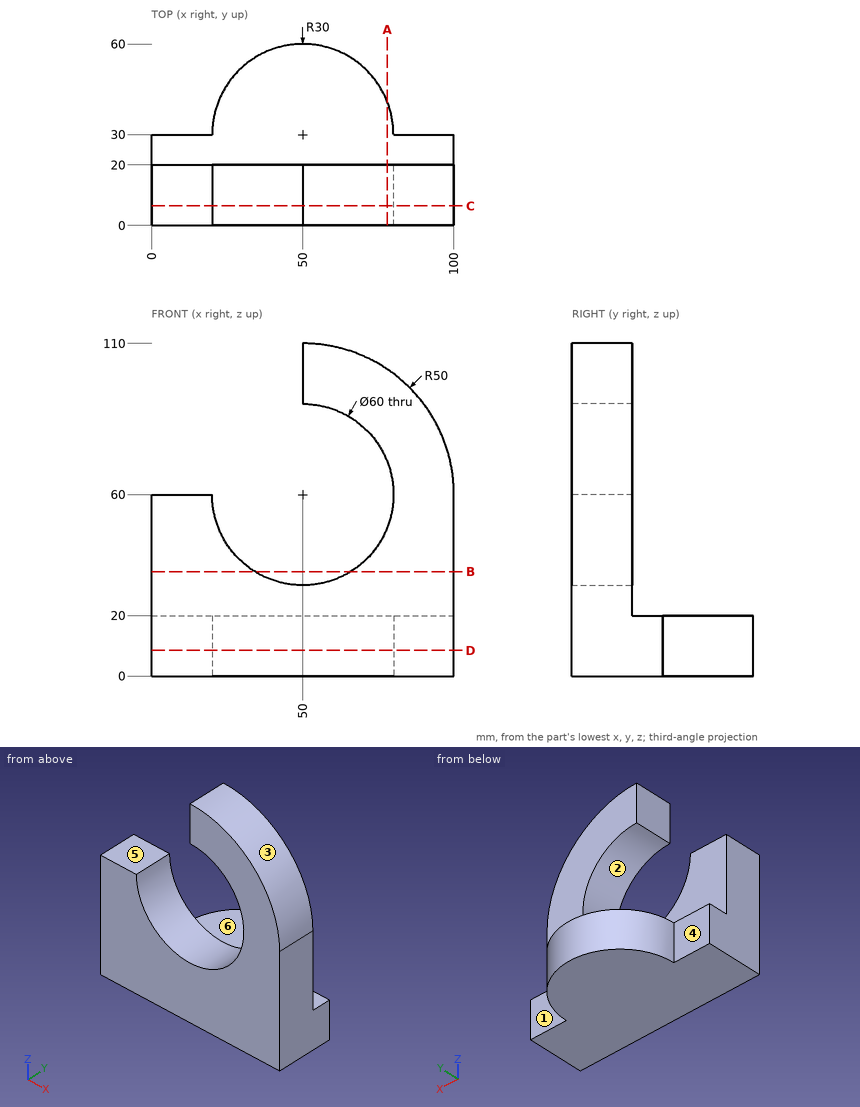
Can you work these out from the drawing? Everything is in mm from the part's minimum corner. A direction names the side the tool comes from. Give positions to 0.01 mm unless a question says otherwise; leave off trailing zeros. Order: outer loops, then holes, each group sorted by start corner. A loop starts at its lowest first (then second) coordinate and runs counter-clockwise, first axis right, second up. Notation, with made-up numbers: M 39,62 L 65,62 A31 ccw 65,93 Z; hole C -12.75,58 d1. An arc over 180 degrees is marked long. Use a Markdown table: item, result. Add a question column.
1. If we mould it in two halves opening along Z, with no side actions, what happens to the marked faces 1, 2 and 3? For each: +Z half, -Z half, draft (parallel to the pull), parting line (faces both ways), or undercut.
2. I need wall thicknesses on probe 1 along Y at (x, z) = (91.5, 83); probe 2 along Z at (x, y) = (74, 5.5). Which ranges of each line are inside material? Lowest first, please. Write a range as from..to.
3. Suppose I cut it at C-C (y = 6.5). List the corners of the cut face in (x, z) for me, and give its area (3 significant figures).
4. Suppose I cut it at B-B (z = 34.5). List the corners of the cut face in (x, y) for me.
5. Suppose I cut it at A-A (x = 78). List the corners of the cut face in (y, z) for me, and give its area (3 significant figures).
6. For pin 1 Ø1 at (x, y) = (37, 15.5) entering from -Z; pin 2 Ø3 at (x, z) = (16, 28) entering from +Y; pin 3 Ø2 at (y, z) = (15, 79.5) entering from -X; pin 4 Ø5 at (y, z) = (13, 94) entering from +X, each with a flat end and sliding along its axis, tell me the tip position at first contact or that it passes through.
7. Suppose I cut it at D-D (z = 8.5). List the corners of the cut face in (x, y) for me.
8. On a 3-axis mill with a long thin cutter (end or side, diameter ignored), from which of +Z, -Z, +X, -X, +Y, -Y can I reach the whole of each face in a straight line? I mean the marked faces 4, 5 and 6. Say none if no direction works.
Results list:
| question | item | result |
|---|---|---|
| 1 | face 1 | draft |
| 1 | face 2 | undercut |
| 1 | face 3 | +Z half |
| 2 | probe 1 | y = 0..20 |
| 2 | probe 2 | z = 0..42, 78..103.86 |
| 3 | outline | M 0,0 L 100,0 L 100,60 A50 ccw 50,110 L 50,90 A30 cw long 20,60 L 0,60 Z |
| 3 | area | 5,840 mm² |
| 4 | outline | M 0,0 L 34.2,0 L 34.2,20 L 0,20 Z; M 65.8,0 L 100,0 L 100,20 L 65.8,20 Z |
| 5 | outline | M 0,0 L 40.77,0 L 40.77,20 L 20,20 L 20,49.23 L 0,49.23 Z; M 0,70.77 L 20,70.77 L 20,101.42 L 0,101.42 Z |
| 5 | area | 2,010 mm² |
| 6 | pin 1 | stops at z = 0 |
| 6 | pin 2 | stops at y = 20 |
| 6 | pin 3 | stops at x = 71.9 |
| 6 | pin 4 | stops at x = 88.83 |
| 7 | outline | M 0,0 L 100,0 L 100,30 L 80,30 A30 ccw 20,30 L 0,30 Z |
| 8 | face 4 | +Z, -Z, -X, +Y |
| 8 | face 5 | +Z, -X, +Y, -Y |
| 8 | face 6 | +Z, +X, -X, +Y |
